```python
from build123d import *

# Parameters (mm, degrees)
F0_W     = 8
F0_H     = 30
F0_R     = 1.5
F1_DEPTH = 25
F0_W_2   = 12
F2_DEPTH = 12
F3_R     = 3.208218
F4_DEPTH = 333


with BuildPart() as f1:
    # F0 (on Front) → F1 (new body)
    with BuildSketch(Plane.XZ):
        with Locations((-22.408133, -12.958233)):
            Rectangle(F0_W, F0_H)
        with Locations((-22.408133, -2.958233)):
            Circle(F0_R, mode=Mode.SUBTRACT)
    extrude(amount=F1_DEPTH)

    # F0 (on Front) → F2 (join)
    with BuildSketch(Plane.XZ):
        with Locations((-12.408133, -12.958233)):
            Rectangle(F0_W_2, F0_H)
    extrude(amount=F2_DEPTH)

    # F3 (on face) → F4 (cut)
    with BuildSketch(Plane.XY.offset(2.041767)):
        with Locations((-21.514958, -4.940173)):
            Circle(F3_R)
    extrude(amount=-F4_DEPTH, mode=Mode.SUBTRACT)


solid = f1.part
```
Can you work these out from the model? Positions are in its coordinate system, mm. A direction names the side the tool comes from. Coordinates: 2 decimals unless noted, no trailing zeros. Loops run counter-clockwise (first coordinate to the right, second up) from the corner with the lowest first, then second, coordinate; pieces in that order, holes last.
Item 1: Suppose I cut it at D-D (y = -22.5). Please give me the cut outline in (x, z).
Answers below:
outline: (-26.41, -27.96) - (-18.41, -27.96) - (-18.41, 2.04) - (-26.41, 2.04) - close; hole circle Ø3 at (-22.41, -2.96)
Item 2: Please list where these lines run through material, in increasing order: L1, parallel to Y at x = -21.5, z = -9; L2, parallel to Y at x = -9.5, z = -1; L3, parallel to Z at x = -21.75, y = -10.5.
Answers below:
L1: y = -25 to -8.15, -1.73 to 0
L2: y = -12 to 0
L3: z = -27.96 to -4.31, -1.61 to 2.04
Item 3: Suppose I cut it at C-C (y = -3.5). Please give me the cut outline in (x, z).
Answers below:
outline: (-26.41, -27.96) - (-24.38, -27.96) - (-24.38, 2.04) - (-26.41, 2.04) - close; (-18.65, -27.96) - (-6.41, -27.96) - (-6.41, 2.04) - (-18.65, 2.04) - close
Item 4: I'm going to push flat-ended pins straight in: pin 1 (1.5 mm diameter, centred on x = -9.5, z = -22, fed in from -Y); pin 2 (12 mm diameter, centred on x = -18.5, z = -24, fed in from +Y); pin 3 (2.5 mm diameter, centred on x = -22.41, z = -2.96, fed in from +Y) (1 decimal); pin 4 (10.5 mm diameter, centred on y = -18, z = -15, fed in from +X). Where does each tip first touch, or does it pass through?
Answers below:
pin 1: stops at y = -12
pin 2: stops at y = 0
pin 3: passes through
pin 4: stops at x = -18.41
Item 5: If we mould it in two halves opening along X, with no side actions, what happens to faces 3 (the face through (-23.907, -1.071, -2.892)), 4 (the face through (-22, -25, -13)), 5 (the face through (-18.408, -18, -13))? For each: released by +X, released by -X, zero draft, split by the parting line, or undercut.
Answers below:
face 3: undercut
face 4: zero draft
face 5: released by +X
Item 6: Which directions (+Z, -Z, +X, -X, +Y, -Y) give clear straight access to the entire face, cutting with the end or side of a thin tool? Please do faces 1 (the face through (-23.6, -15.91, -3.87)), 2 (the face through (-12, -12, -13)).
Answers below:
face 1: +Y, -Y
face 2: +Z, -Z, +X, -Y
Item 7: Suppose I cut it at A-A (x = -20.25). Please give me the cut outline in (y, z).
Answers below:
outline: (-25, -27.96) - (-7.89, -27.96) - (-7.89, 2.04) - (-25, 2.04) - close; (-1.99, -27.96) - (0, -27.96) - (0, 2.04) - (-1.99, 2.04) - close
Item 8: Suppose I cut it at B-B (z = -0.5). Please give me the cut outline in (x, y).
Answers below:
outline: (-26.41, -25) - (-18.41, -25) - (-18.41, -12) - (-6.41, -12) - (-6.41, 0) - (-26.41, 0) - close; hole circle Ø6.42 at (-21.51, -4.94)
